Input: part model. Units: mm. Frame: model coordinates. A direction names the side the tool comes from. Coordinates: 2 decimals unless noted, no trailing zeros. Write each loop counter-clockwise with the first axis right and the second up, starting at its lowest first coordinate (ties: lowest second). Pieces come first, ordered by that corner, then holes. Notation, with made-up numbers: M 44,-36.75 L 54,-36.75 A31 ccw 54,-6.75 Z; hole C 15.5,21.5 d2. An arc over 180 degrees is marked long. Use CSV: the item, a comma, the result in double quotes.
```python
from build123d import *

# Parameters (mm, degrees)
F1_DEPTH = 25.4


with BuildPart() as f1:
    # F0 (on Front) → F1 (new body)
    with BuildSketch(Plane.XZ):
        with BuildLine():
            Line((90.424, 208.28), (-90.424, 208.28))
            Line((-90.424, 208.28), (-90.424, 190.119))
            Line((-90.424, 190.119), (-21.336, 190.119))
            ThreePointArc((-21.336, 190.119), (-10.11068, 185.46932), (-5.461, 174.244))
            Line((-5.461, 174.244), (-5.461, -174.244))
            ThreePointArc((-5.461, -174.244), (-10.11068, -185.46932), (-21.336, -190.119))
            Line((-21.336, -190.119), (-90.424, -190.119))
            Line((-90.424, -190.119), (-90.424, -208.28))
            Line((-90.424, -208.28), (90.424, -208.28))
            Line((90.424, -208.28), (90.424, -190.119))
            Line((90.424, -190.119), (21.336, -190.119))
            ThreePointArc((21.336, -190.119), (10.11068, -185.46932), (5.461, -174.244))
            Line((5.461, -174.244), (5.461, 174.244))
            ThreePointArc((5.461, 174.244), (10.11068, 185.46932), (21.336, 190.119))
            Line((21.336, 190.119), (90.424, 190.119))
            Line((90.424, 190.119), (90.424, 208.28))
        make_face()
    extrude(amount=F1_DEPTH)


solid = f1.part
```
1. Mould query, pull axis Z, two halves, no side actions, for faces 4 (the cylindrical face through (10.23, -12.52, -185.59)), 5 (the flat face through (90.424, -13, -199)), 6 (the flat face through (-1, -13, -208.28)). Classes: pulls with the +Z half, pulls with the -Z half, needs draft (parallel to the pull), parting line crosses it, or undercut.
Resolved:
face 4,"undercut"
face 5,"needs draft"
face 6,"pulls with the -Z half"
2. Access query for faces 1 (the flat face through (1, -13, 208.28)), 2 (the flat face through (-56, -13, 190.119)), 3 (the cylindrical face through (9.99, -12.52, 185.35)). Directions: +Z, -Z, +X, -X, +Y, -Y. A direction counts if a zero-diameter tool reaches every point of the face in a straight line with its end or side. Return the directions, or none.
Resolved:
face 1,"+Z, +X, -X, +Y, -Y"
face 2,"-X, +Y, -Y"
face 3,"+X, +Y, -Y"
3. Section A-A (x = -57). Return loops of the section in (y, z).
Resolved:
outline,"M -25.4,-208.28 L 0,-208.28 L 0,-190.12 L -25.4,-190.12 Z; M -25.4,190.12 L 0,190.12 L 0,208.28 L -25.4,208.28 Z"
4. Section B-B (y = -14.75). Return loops of the section in (x, z) (3 decimals).
Resolved:
outline,"M -90.424,-208.28 L 90.424,-208.28 L 90.424,-190.119 L 21.336,-190.119 A15.875 cw 5.461,-174.244 L 5.461,174.244 A15.875 cw 21.336,190.119 L 90.424,190.119 L 90.424,208.28 L -90.424,208.28 L -90.424,190.119 L -21.336,190.119 A15.875 cw -5.461,174.244 L -5.461,-174.244 A15.875 cw -21.336,-190.119 L -90.424,-190.119 Z"
5. Contact query for a flat-ended pin moving along its axis: pin 1 Ø1.5 at (y, z) = (-3.5, 96.5) entering from -X. Output: stop coordinate, or through.
Resolved:
pin 1,"stops at x = -5.46"
6. Material intervals for line 1 (Z direction, x = -40.5, y = -6); line 2 (X direction, y = -12, z = -172); line 3 (Z direction, x = 10, y = -8.75), sorted ascending. Write a range as [from, to].
Resolved:
line 1,"z = [-208.28, -190.12], [190.12, 208.28]"
line 2,"x = [-5.46, 5.46]"
line 3,"z = [-208.28, -185.36], [185.36, 208.28]"
7. Section C-C (z = 89). Return loops of the section in (x, y).
Resolved:
outline,"M -5.46,-25.4 L 5.46,-25.4 L 5.46,0 L -5.46,0 Z"
